Source: CAD feature listing. Evaluate the final solid. Frame: model axes, mm. A direction names the side the tool comes from. Give positions to 0.01 mm unless a question says otherwise; leave off trailing zeros. Write each loop counter-clockwise with the first axis right and the second up, starting at its lowest first coordinate (ties: lowest second). Pieces come first, ordered by that corner, then holes. Notation, with made-up numbers: M -36,39.5 L 8,39.5 A36 ccw 8,76.5 Z; hole C 36,-12.5 d8. An arc over 180 degrees is marked long. Answer as a JSON object with one key per item and string values. Group by question number.
```python
from build123d import *

# Parameters (mm, degrees)
BOSS_EXTRUDE1_DEPTH = 82
SKETCH3_R           = 7.537472245
CUT_EXTRUDE2_DEPTH  = 11
SKETCH4_R           = 6.5
CUT_EXTRUDE3_DEPTH  = 11


with BuildPart() as part:
    # Sketch1 → Boss-Extrude1 (new body)
    with BuildSketch(Plane.XY):
        with BuildLine():
            Line((33.003348812, 0), (33.003348812, -33.227979662))
            Line((33.003348812, -33.227979662), (65.632108119, -33.227979662))
            Line((65.632108119, -33.227979662), (65.632108119, -23.227979662))
            Line((65.632108119, -23.227979662), (43.003348812, -23.227979662))
            Line((43.003348812, -23.227979662), (43.003348812, -2.369569967))
            ThreePointArc((43.003348812, -2.369569967), (20.809611253, 35.186501293), (-22.793831907, 33.859768466))
            Line((-22.793831907, 33.859768466), (-23.793831907, 33.859768466))
            Line((-23.793831907, 33.859768466), (-23.793831907, 59.275147612))
            Line((-23.793831907, 59.275147612), (-33.793831907, 59.275147612))
            Line((-33.793831907, 59.275147612), (-33.793831907, 23.859768466))
            Line((-33.793831907, 23.859768466), (-22.793831907, 23.859768466))
            ThreePointArc((-22.793831907, 23.859768466), (12.978190551, 30.342272193), (33.003348812, 0))
        make_face()
    extrude(amount=-BOSS_EXTRUDE1_DEPTH)

    # Sketch3 → Cut-Extrude2 (cut, through all)
    with BuildSketch(Plane(origin=(0, -23.227979662, 0), x_dir=(1, 0, 0), z_dir=(0, 1, 0))):
        with Locations((54.317728466, 16)):
            Circle(SKETCH3_R)
        with Locations((54.317728466, 66)):
            Circle(SKETCH3_R)
    extrude(amount=-CUT_EXTRUDE2_DEPTH, mode=Mode.SUBTRACT)

    # Sketch4 → Cut-Extrude3 (cut, through all)
    with BuildSketch(Plane(origin=(-23.793831907, 0, 0), x_dir=(0, 0, -1), z_dir=(1, 0, 0))):
        with Locations((16.5, 46.567458039)):
            Circle(SKETCH4_R)
        with Locations((65.5, 46.567458039)):
            Circle(SKETCH4_R)
    extrude(amount=-CUT_EXTRUDE3_DEPTH, mode=Mode.SUBTRACT)


solid = part.part
```
(1) Ray query, L1, parallel to X at y = -27.25, z = -16; L2, parallel to X at y = -4.5, z = -66; L3, parallel to Y at x = 56.5, z = -31. Return the intervals inside material, ascending. Write a range as [from, to].
(2) Section D-D, the plane x = 37. Return loops of the section in (y, z).
(3) Section A-A, the plane z = -66. Return loops of the section in (x, y).
(4) Section C-C, the plane z = -76. Return loops of the section in (x, y), plus the area to 3 significant figures.
(5) Section B-B, the plane y = 37. Return loops of the section in (x, z).
(6) Contact query for flat-ended pins moving along their axis: pin 1 Ø11.5 at (x, z) = (59.5, -34) entering from +Y; pin 2 Ø21 at (y, z) = (46.57, -65.5) entering from +X; pin 3 Ø9 at (x, z) = (-27.5, -29.5) entering from -Y. Output: stop coordinate, or through.
(7) Pull-direction query (Z, two-part tool) for faces 6 (the cylindrical face through (58.37, -28.158, -72.356)), 7 (the flat face through (27, 20, 0)), 8 (the flat face through (49, -33.228, -40)); classes: pulls with the +Z half, pulls with the -Z half, needs draft (parallel to the pull), parting line crosses it, or undercut.
(8) Access query for faces 1 (the flat face through (65.632, -28, -40)), 2 (the flat face through (43.003, -13, -40)), 3 (the flat face through (-28, 23.86, -40)), 4 (the flat face through (-33.794, 42, -40)), 5 (the flat face through (-23.794, 46, -40)). Directions: +Z, -Z, +X, -X, +Y, -Y. A direction counts if a zero-diameter tool reaches every point of the face in a straight line with its end or side. Return the directions, or none.
Reported:
{
 "1": {"L1": "x = [33, 46.78], [61.86, 65.63]", "L2": "x = [33, 43]", "L3": "y = [-33.23, -23.23]"},
 "2": {"outline": "M -33.23,-82 L 19.51,-82 L 19.51,0 L -33.23,0 Z"},
 "3": {"outline": "M -33.79,23.86 L -22.79,23.86 A33 cw 33,0 L 33,-33.23 L 46.78,-33.23 L 46.78,-23.23 L 43,-23.23 L 43,-2.37 A42.87 ccw -22.79,33.86 L -23.79,33.86 L -23.79,40.09 L -33.79,40.09 Z; M -33.79,53.05 L -23.79,53.05 L -23.79,59.28 L -33.79,59.28 Z; M 61.86,-33.23 L 65.63,-33.23 L 65.63,-23.23 L 61.86,-23.23 Z"},
 "4": {"outline": "M -33.79,23.86 L -22.79,23.86 A33 cw 33,0 L 33,-33.23 L 65.63,-33.23 L 65.63,-23.23 L 43,-23.23 L 43,-2.37 A42.87 ccw -22.79,33.86 L -23.79,33.86 L -23.79,59.28 L -33.79,59.28 Z", "area": "1,600 mm2"},
 "5": {"outline": "M -33.79,-82 L -23.79,-82 L -23.79,0 L -33.79,0 Z; M -16.84,-82 L 17.1,-82 L 17.1,0 L -16.84,0 Z"},
 "6": {"pin 1": "stops at y = -23.23", "pin 2": "stops at x = 19.12", "pin 3": "stops at y = 23.86"},
 "7": {"face 6": "undercut", "face 7": "pulls with the +Z half", "face 8": "needs draft"},
 "8": {"face 1": "+Z, -Z, +X, +Y, -Y", "face 2": "+Z, -Z, +X, +Y", "face 3": "+Z, -Z, -X, -Y", "face 4": "+Z, -Z, -X, +Y, -Y", "face 5": "+Z, -Z, +Y"}
}
